```python
from build123d import *

# Parameters (mm, degrees)
SKETCH1_R           = 4
BOSS_EXTRUDE2_DEPTH = 10
FILLET1_R           = 30
FILLET2_R           = 30


with BuildPart() as part:
    # Sketch1 → Boss-Extrude2 (new body)
    with BuildSketch(Plane(origin=(0, 0, 0), x_dir=(1, 0, 0), z_dir=(0, 1, 0))):
        Polygon((12.5, -12.5), (46.843467743, 0), (248.156532257, 0), (282.5, -12.5), (307.5, -12.5), (341.843467743, 0), (543.156532257, 0), (577.5, -12.5), (590, -12.5), (590, 40), (0, 40), (0, -12.5), align=None)
        with Locations(Location((12.5, 2.5, 0), (0, 0, 270))):
            Circle(SKETCH1_R, mode=Mode.SUBTRACT)
        with Locations(Location((282.5, 2.5, 0), (0, 0, 270))):
            Circle(SKETCH1_R, mode=Mode.SUBTRACT)
        with Locations(Location((307.5, 2.5, 0), (0, 0, 270))):
            Circle(SKETCH1_R, mode=Mode.SUBTRACT)
        with Locations(Location((577.5, 2.5, 0), (0, 0, 270))):
            Circle(SKETCH1_R, mode=Mode.SUBTRACT)
    extrude(amount=BOSS_EXTRUDE2_DEPTH)

    # Fillet1
    fillet1_edges = [part.edges().sort_by_distance(p)[0] for p in [
        (46.843467743, 5, 0),
        (12.5, 5, 12.5),
    ]]
    fillet(fillet1_edges, radius=FILLET1_R)

    # Fillet2
    fillet2_edges = [part.edges().sort_by_distance(p)[0] for p in [
        (307.5, 5, 12.5),
        (282.5, 5, 12.5),
        (248.156532257, 5, 0),
        (577.5, 5, 12.5),
        (543.156532257, 5, 0),
        (341.843467743, 5, 0),
    ]]
    fillet(fillet2_edges, radius=FILLET2_R)


solid = part.part
```
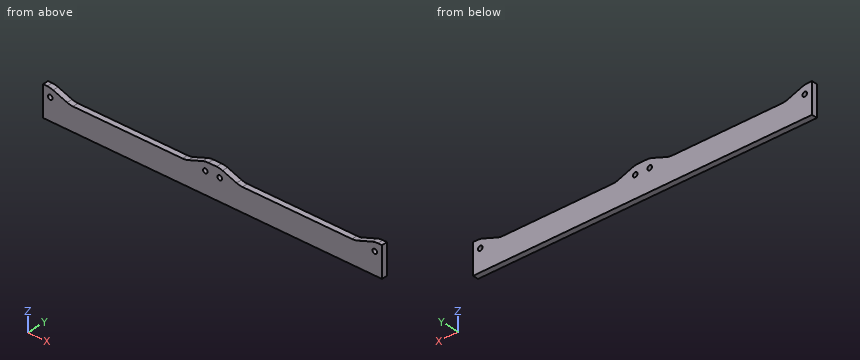
Here's how the part is built. I have some questions about the finished solid (model axes, mm). Round coordinates to 2 decimals unless told otherwise and drop trailing zeros. Order: outer loops, then holes, each group sorted by start corner. A loop starts at its lowest first (then second) coordinate and runs counter-clockwise, first axis right, second up. Notation, with made-up numbers: M 0.25,-29.75 L 58.25,-29.75 A11 cw 58.25,-18.75 Z; hole C -9.75,57.5 d3. An arc over 180 degrees is marked long. Answer as CSV lines item,"result".
Item 1: Imagine slicing it at C-C on x = 320. List the corners of the cut face in (y, z) for me.
From the geometry:
outline,"M 0,-40 L 10,-40 L 10,7.95 L 0,7.95 Z"
Item 2: Please list where these lines run through material, in increasing order: L1, parallel to X at y = 2.75, z = -2.5; L2, parallel to Z at x = 182, y = 4.75; L3, parallel to Z at x = 304.5, y = 3.75. Write a range as [from, to].
From the geometry:
L1,"[0, 8.5], [16.5, 278.5], [286.5, 303.5], [311.5, 573.5], [581.5, 590]"
L2,"[-40, 0]"
L3,"[-40, -5.15], [0.15, 12.41]"
Item 3: Imagine slicing it at B-B on x = 389. List the corners of the cut face in (y, z) for me, and give its area (3 significant figures).
From the geometry:
outline,"M 0,-40 L 10,-40 L 10,0 L 0,0 Z"
area,"400 mm2"
Item 4: For pin 1 (5 mm diameter, centred on x = 73, y = 7.5, fed in from +Z), with a flat end and sliding along its axis, tell me the tip position at first contact or that it passes through.
From the geometry:
pin 1,"z = 0"
Item 5: Imagine slicing it at A-A on y = 3. List the corners of the cut face in (x, z) for me.
From the geometry:
outline,"M 0,-40 L 590,-40 L 590,12.5 L 582.79,12.5 A30 ccw 572.53,10.69 L 548.13,1.81 A30 cw 537.87,0 L 347.13,0 A30 cw 336.87,1.81 L 312.47,10.69 A30 ccw 302.21,12.5 L 287.79,12.5 A30 ccw 277.53,10.69 L 253.13,1.81 A30 cw 242.87,0 L 52.13,0 A30 cw 41.87,1.81 L 17.47,10.69 A30 ccw 7.21,12.5 L 0,12.5 Z; hole C 12.5,-2.5 d8; hole C 282.5,-2.5 d8; hole C 307.5,-2.5 d8; hole C 577.5,-2.5 d8"
